For this review, take the finished solid that the model builds, in its own axes (mm). Give positions to 0.01 mm unless a question says otherwise; leave off trailing zeros. Write each loop counter-clockwise with the first axis right and the second up, starting at its lowest first coordinate (ties: lowest second). Pieces come first, ordered by that corner, then holes.
1) Draft analysis for pull direction X (two halves, no side actions). For faces 1 (the face through (-2, -21, 93)), 2 (the face through (-117, -18, 266)), 3 (the face through (146.99, -18.46, -117.15)), state which applies: pulls with the +X half, pulls with the -X half, needs draft (parallel to the pull), parting line crosses it, or undercut.
2) For P1, Ø6, axis at x = 120, z = -90, coming from the -Y side, flat-tipped, find the tip position at first contact; note if it passes through.
3) Wall thickness on line 1 along X through (y, z) = (-18.7, -90); line 2 along X through (y, z) = (-19.6, -51.5); line 3 along Z through (x, y) = (-120, -18.8): over which ranges is each line inside the solid? List them lowest first.
4) We need section A-A on x = 120. Give the boundary of the cut face in (y, z).
from build123d import *

# Parameters (mm, degrees)
SKIZZE2_W                            = 300
SKIZZE2_H                            = 5
AUFSATZ_LINEAR_AUSTRAGEN1_DEPTH      = 300
AUFSATZ_LINEAR_AUSTRAGEN1_DEPTH_BACK = 120
SCHNITT_LINEAR_AUSTRAGEN1_DEPTH      = 5
SKIZZE6_R                            = 3
SCHNITT_LINEAR_AUSTRAGEN2_DEPTH      = 5
SKIZZE8_R                            = 5
SCHNITT_LINEAR_AUSTRAGEN3_DEPTH      = 21
VERRUNDUNG1_R                        = 10
SKIZZE9_R                            = 2.1
SCHNITT_LINEAR_AUSTRAGEN4_DEPTH      = 5


with BuildPart() as part:
    # Skizze2 → Aufsatz-Linear austragen1 (new body, two sides)
    with BuildSketch(Plane.XY) as aufsatz_linear_austragen1_sk:
        with Locations((0, -18.5)):
            Rectangle(SKIZZE2_W, SKIZZE2_H)
    extrude(amount=AUFSATZ_LINEAR_AUSTRAGEN1_DEPTH)
    extrude(aufsatz_linear_austragen1_sk.sketch, amount=-AUFSATZ_LINEAR_AUSTRAGEN1_DEPTH_BACK)

    # Skizze4 → Schnitt-Linear austragen1 (cut)
    with BuildSketch(Plane(origin=(0, -16, 0), x_dir=(1, 0, 0), z_dir=(0, 1, 0))):
        with BuildLine():
            Line((-19, -121), (-19, -99))
            ThreePointArc((-19, -99), (-15, -95), (-11, -99))
            Line((-11, -99), (-11, -121))
            ThreePointArc((-11, -121), (-15, -125), (-19, -121))
        make_face()
        with BuildLine():
            Line((19, -121), (19, -99))
            ThreePointArc((19, -99), (15, -95), (11, -99))
            Line((11, -99), (11, -121))
            ThreePointArc((11, -121), (15, -125), (19, -121))
        make_face()
        with BuildLine():
            Line((-19, -259), (-19, -281))
            ThreePointArc((-19, -281), (-15, -285), (-11, -281))
            Line((-11, -281), (-11, -259))
            ThreePointArc((-11, -259), (-15, -255), (-19, -259))
        make_face()
        with BuildLine():
            Line((19, -259), (19, -281))
            ThreePointArc((19, -281), (15, -285), (11, -281))
            Line((11, -281), (11, -259))
            ThreePointArc((11, -259), (15, -255), (19, -259))
        make_face()
    extrude(amount=-SCHNITT_LINEAR_AUSTRAGEN1_DEPTH, mode=Mode.SUBTRACT)

    # Skizze6 → Schnitt-Linear austragen2 (cut)
    with BuildSketch(Plane(origin=(0, -16, 0), x_dir=(1, 0, 0), z_dir=(0, 1, 0))):
        with Locations((-53, 7.5)):
            Circle(SKIZZE6_R)
        with Locations((-53, -7.5)):
            Circle(SKIZZE6_R)
    extrude(amount=-SCHNITT_LINEAR_AUSTRAGEN2_DEPTH, mode=Mode.SUBTRACT)

    # Skizze8 → Schnitt-Linear austragen3 (cut)
    with BuildSketch(Plane(origin=(0, 0, 0), x_dir=(1, 0, 0), z_dir=(0, 1, 0))):
        with Locations((-120, 90)):
            Circle(SKIZZE8_R)
        with Locations((120, 90)):
            Circle(SKIZZE8_R)
        with Locations((120, -270)):
            Circle(SKIZZE8_R)
        with Locations((-120, -270)):
            Circle(SKIZZE8_R)
    extrude(amount=-SCHNITT_LINEAR_AUSTRAGEN3_DEPTH, mode=Mode.SUBTRACT)

    # Verrundung1
    verrundung1_edges = [part.edges().sort_by_distance(p)[0] for p in [
        (-150, -18.5, -120),
        (150, -18.5, -120),
        (150, -18.5, 300),
        (-150, -18.5, 300),
    ]]
    fillet(verrundung1_edges, radius=VERRUNDUNG1_R)

    # Skizze9 → Schnitt-Linear austragen4 (cut)
    with BuildSketch(Plane(origin=(0, -16, 0), x_dir=(1, 0, 0), z_dir=(0, 1, 0))):
        with Locations((75.5, 51.5)):
            Circle(SKIZZE9_R)
        with Locations((-75.5, 51.5)):
            Circle(SKIZZE9_R)
    extrude(amount=-SCHNITT_LINEAR_AUSTRAGEN4_DEPTH, mode=Mode.SUBTRACT)


solid = part.part
Results list:
1. face 1: needs draft
1. face 2: undercut
1. face 3: pulls with the +X half
2. P1: passes through
3. line 1: x = -150 to -125, -115 to 115, 125 to 150
3. line 2: x = -150 to -77.6, -73.4 to 73.4, 77.6 to 150
3. line 3: z = -120 to -95, -85 to 265, 275 to 300
4. outline: (-21, -120) - (-16, -120) - (-16, -95) - (-21, -95) - close; (-21, -85) - (-16, -85) - (-16, 265) - (-21, 265) - close; (-21, 275) - (-16, 275) - (-16, 300) - (-21, 300) - close
